```python
from build123d import *

# Parameters (mm, degrees)
F0_R     = 1.75
F0_R_2   = 8.25
F1_DEPTH = 3.2
F2_R     = 9.525
F3_DEPTH = 1.95
F4_R     = 10.75
F4_R_2   = 9.525
F5_DEPTH = 2
F6_R     = 2
F7_R     = 3


with BuildPart() as f1:
    # F0 (on Top) → F1 (new body)
    with BuildSketch(Plane.XY):
        with BuildLine():
            Line((14.65, -10.15), (10.431534, -5.931534))
            ThreePointArc((10.431534, -5.931534), (12, 0), (10.431534, 5.931534))
            Line((10.431534, 5.931534), (14.65, 10.15))
            Line((14.65, 10.15), (16.65, 10.15))
            Line((16.65, 10.15), (16.65, 16.65))
            Line((16.65, 16.65), (10.15, 16.65))
            Line((10.15, 16.65), (10.15, 14.65))
            Line((10.15, 14.65), (5.983453, 10.483453))
            ThreePointArc((5.983453, 10.483453), (0, 12.070812), (-5.983453, 10.483453))
            Line((-5.983453, 10.483453), (-10.15, 14.65))
            Line((-10.15, 14.65), (-10.15, 16.65))
            Line((-10.15, 16.65), (-16.65, 16.65))
            Line((-16.65, 16.65), (-16.65, 10.15))
            Line((-16.65, 10.15), (-14.65, 10.15))
            Line((-14.65, 10.15), (-10.431534, 5.931534))
            ThreePointArc((-10.431534, 5.931534), (-12, 0), (-10.431534, -5.931534))
            Line((-10.431534, -5.931534), (-14.65, -10.15))
            Line((-14.65, -10.15), (-16.65, -10.15))
            Line((-16.65, -10.15), (-16.65, -16.65))
            Line((-16.65, -16.65), (-10.15, -16.65))
            Line((-10.15, -16.65), (-10.15, -14.65))
            Line((-10.15, -14.65), (-5.983453, -10.483453))
            ThreePointArc((-5.983453, -10.483453), (0, -12.070812), (5.983453, -10.483453))
            Line((5.983453, -10.483453), (10.15, -14.65))
            Line((10.15, -14.65), (10.15, -16.65))
            Line((10.15, -16.65), (16.65, -16.65))
            Line((16.65, -16.65), (16.65, -10.15))
            Line((16.65, -10.15), (14.65, -10.15))
        make_face()
        with Locations((-13.4, -13.4)):
            Circle(F0_R, mode=Mode.SUBTRACT)
        with Locations((13.4, -13.4)):
            Circle(F0_R, mode=Mode.SUBTRACT)
        with Locations((-13.4, 13.4)):
            Circle(F0_R, mode=Mode.SUBTRACT)
        Circle(F0_R_2, mode=Mode.SUBTRACT)
        with Locations((13.4, 13.4)):
            Circle(F0_R, mode=Mode.SUBTRACT)
    extrude(amount=F1_DEPTH)

    # F2 (on face) → F3 (cut)
    with BuildSketch(Plane.XY.offset(3.2)):
        Circle(F2_R)
    extrude(amount=-F3_DEPTH, mode=Mode.SUBTRACT)

    # F4 (on face) → F5 (join)
    with BuildSketch(Plane.XY.offset(3.2)):
        Circle(F4_R)
        Circle(F4_R_2, mode=Mode.SUBTRACT)
    extrude(amount=F5_DEPTH)

    # F6
    f6_edges = [f1.edges().sort_by_distance(p)[0] for p in [
        (-14.65, 10.15, 1.6),
        (-10.15, 14.65, 1.6),
        (10.15, 14.65, 1.6),
        (14.65, 10.15, 1.6),
        (14.65, -10.15, 1.6),
        (10.15, -14.65, 1.6),
        (-10.15, -14.65, 1.6),
        (-14.65, -10.15, 1.6),
    ]]
    fillet(f6_edges, radius=F6_R)

    # F7
    f7_edges = [f1.edges().sort_by_distance(p)[0] for p in [
        (-10.431534, -5.931534, 1.6),
        (-10.431534, 5.931534, 1.6),
        (-5.983453, 10.483453, 1.6),
        (5.983453, 10.483453, 1.6),
        (10.431534, 5.931534, 1.6),
        (10.431534, -5.931534, 1.6),
        (-5.983453, -10.483453, 1.6),
        (5.983453, -10.483453, 1.6),
    ]]
    fillet(f7_edges, radius=F7_R)


solid = f1.part
```
Here's how the part is built. I have some questions about the finished solid (model axes, mm). A direction names the side the tool comes from. Round coordinates to 2 decimals unless told otherwise and drop trailing zeros. Write each loop counter-clockwise with the first axis right and the second up, starting at its lowest first coordinate (ties: lowest second). Pieces come first, ordered by that corner, then holes.
Q1. Which directions (+Z, -Z, +X, -X, +Y, -Y) give clear straight access to the entire face, cutting with the end or side of a thin tool? Please do faces 1 (the flat face through (-16, 10.15, 2)), 2 (the flat face through (-3, 8, 1.25)), 3 (the flat face through (-10.15, -16, 2)), 4 (the flat face through (13, -8.5, 1.6)), 5 (the flat face through (10.15, 16, 2)).
Q2. If we mould it in two halves opening along X, with no side actions, what happens to faces 6 (the flat face through (16, 10.15, 2)), 7 (the cylindrical face through (9.994, 14.703, 1.622)), 8 (the flat face through (-16.65, 13, 2))? For each: +X half, -X half, draft (parallel to the pull), parting line (faces both ways), or undercut.
Q3. Please list where these lines run through material, in increasing order: probe 1 along X at (y, z) = (0, 0.3); probe 2 along Y at (x, z) = (-13.4, 0.75); probe 3 along X at (y, z) = (13.5, 2.7).
Q4. If we section it at D-D on y = 1.5: Write out the boundary of the cut face in (x, z).
Q5. If we section it at C-C on x = 0: Write out the boundary of the cut face in (y, z) (3 decimals), plus the area to 3 significant figures.
Q6. If we section it at A-A on y = 13.4: Write out the boundary of the cut face in (x, z).
Q7. Will these pins go through, and if not, where does the flat tip stop? P1, Ø6, axis at x = 12, y = -7.5, coming from the +Z side; P2, Ø2, axis at y = -1.5, z = 0.5, coming from the -X side.
Answer below:
1. face 1: +Z, -Z, -X
1. face 2: +Z
1. face 3: +Z, -Z, -Y
1. face 4: +Z, -Z, +X
1. face 5: +Z, -Z, +Y
2. face 6: draft
2. face 7: undercut
2. face 8: -X half
3. probe 1: x = -12 to -8.25, 8.25 to 12
3. probe 2: y = -16.65 to -15.15, -11.65 to -8.9, 8.9 to 11.65, 15.15 to 16.65
3. probe 3: x = -16.65 to -15.15, -11.65 to -9, 9 to 11.65, 15.15 to 16.65
4. outline: (-11.91, 0) - (-8.11, 0) - (-8.11, 1.25) - (-9.41, 1.25) - (-9.41, 5.2) - (-10.64, 5.2) - (-10.64, 3.2) - (-11.91, 3.2) - close; (8.11, 0) - (11.91, 0) - (11.91, 3.2) - (10.64, 3.2) - (10.64, 5.2) - (9.41, 5.2) - (9.41, 1.25) - (8.11, 1.25) - close
5. outline: (-12.071, 0) - (-8.25, 0) - (-8.25, 1.25) - (-9.525, 1.25) - (-9.525, 5.2) - (-10.75, 5.2) - (-10.75, 3.2) - (-12.071, 3.2) - close; (8.25, 0) - (12.071, 0) - (12.071, 3.2) - (10.75, 3.2) - (10.75, 5.2) - (9.525, 5.2) - (9.525, 1.25) - (8.25, 1.25) - close
5. area: 24.4 mm2
6. outline: (-16.65, 0) - (-15.15, 0) - (-15.15, 3.2) - (-16.65, 3.2) - close; (-11.65, 0) - (-8.9, 0) - (-8.9, 3.2) - (-11.65, 3.2) - close; (8.9, 0) - (11.65, 0) - (11.65, 3.2) - (8.9, 3.2) - close; (15.15, 0) - (16.65, 0) - (16.65, 3.2) - (15.15, 3.2) - close
7. P1: stops at z = 3.2
7. P2: stops at x = -11.99
